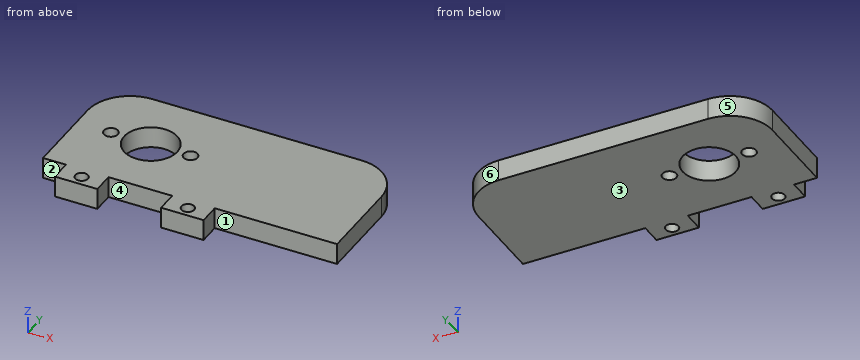
from build123d import *

# Parameters (mm, degrees)
SKETCH2_W                 = 87.884
SKETCH2_H                 = 44.45
BOSS_EXTRUDE1_DEPTH       = 3.175
CUT_EXTRUDE1_REACH        = 51.651
SKETCH3_R                 = 7.9375
F_8_CLEARANCE_HOLE1_D     = 4.1656
CIRPATTERN1_COUNT         = 2
CUT_EXTRUDE2_REACH        = 51.651
SKETCH6_W                 = 6.858
SKETCH6_H                 = 6.35
SKETCH6_W_2               = 19.05
SKETCH6_W_3               = 36.576
F_6_CLEARANCE_HOLE1_D     = 3.7973
F_6_CLEARANCE_HOLE1_DEPTH = 6.35
F_6_CLEARANCE_HOLE1_TIP   = 1.140824014
FILLET1_R                 = 12.7


with BuildPart() as part:
    # Sketch2 → Boss-Extrude1 (new, symmetric)
    with BuildSketch(Plane.XY):
        Rectangle(SKETCH2_W, SKETCH2_H)
    extrude(amount=BOSS_EXTRUDE1_DEPTH, both=True)

    # Sketch3 → Cut-Extrude1 (cut, up to next)
    with BuildSketch(Plane.XY.offset(3.175), mode=Mode.PRIVATE) as cut_extrude1_sk1:
        with Locations((-21.717, 3.175)):
            Circle(SKETCH3_R)
    cut_extrude1_tool1 = extrude(cut_extrude1_sk1.sketch, amount=-CUT_EXTRUDE1_REACH, mode=Mode.PRIVATE) & part.part
    add(cut_extrude1_tool1.solids().sort_by_distance((-21.717, 3.175, 3.175))[0], mode=Mode.SUBTRACT)

    # #8 Clearance Hole1 (through all)
    with Locations(Plane.XY.offset(3.175)):
        with Locations((-33.6169, 3.175)):
            f_8_clearance_hole1 = Hole(F_8_CLEARANCE_HOLE1_D / 2)

    # CirPattern1: #8 Clearance Hole1 ×2 about axis
    cirpattern1_axis = Axis((-21.717, 3.175, 0), (0, 0, 1))
    for i in range(1, CIRPATTERN1_COUNT):
        add(f_8_clearance_hole1.rotate(cirpattern1_axis, i * 360 / CIRPATTERN1_COUNT), mode=Mode.SUBTRACT)

    # Sketch6 → Cut-Extrude2 (cut, up to next)
    with BuildSketch(Plane.XY.offset(3.175), mode=Mode.PRIVATE) as cut_extrude2_sk1:
        with Locations((-40.513, -19.05)):
            Rectangle(SKETCH6_W, SKETCH6_H)
    cut_extrude2_tool1 = extrude(cut_extrude2_sk1.sketch, amount=-CUT_EXTRUDE2_REACH, mode=Mode.PRIVATE) & part.part
    # Sketch6 → Cut-Extrude2 (cut, up to next)
    with BuildSketch(Plane.XY.offset(3.175), mode=Mode.PRIVATE) as cut_extrude2_sk2:
        with Locations((-14.859, -19.05)):
            Rectangle(SKETCH6_W_2, SKETCH6_H)
    cut_extrude2_tool2 = extrude(cut_extrude2_sk2.sketch, amount=-CUT_EXTRUDE2_REACH, mode=Mode.PRIVATE) & part.part
    # Sketch6 → Cut-Extrude2 (cut, up to next)
    with BuildSketch(Plane.XY.offset(3.175), mode=Mode.PRIVATE) as cut_extrude2_sk3:
        with Locations((25.654, -19.05)):
            Rectangle(SKETCH6_W_3, SKETCH6_H)
    cut_extrude2_tool3 = extrude(cut_extrude2_sk3.sketch, amount=-CUT_EXTRUDE2_REACH, mode=Mode.PRIVATE) & part.part
    add(cut_extrude2_tool1.solids().sort_by_distance((-40.513, -19.05, 3.175))[0], mode=Mode.SUBTRACT)
    add(cut_extrude2_tool2.solids().sort_by_distance((-14.859, -19.05, 3.175))[0], mode=Mode.SUBTRACT)
    add(cut_extrude2_tool3.solids().sort_by_distance((25.654, -19.05, 3.175))[0], mode=Mode.SUBTRACT)

    # #6 Clearance Hole1
    with Locations(Plane.XY.offset(3.175)):
        with Locations((1.016, -19.05), (-30.734, -19.05)):
            Hole(F_6_CLEARANCE_HOLE1_D / 2, depth=F_6_CLEARANCE_HOLE1_DEPTH)
            with Locations((0, 0, -(F_6_CLEARANCE_HOLE1_DEPTH + F_6_CLEARANCE_HOLE1_TIP / 2))):  # 118° drill point
                Cone(0, F_6_CLEARANCE_HOLE1_D / 2, F_6_CLEARANCE_HOLE1_TIP, mode=Mode.SUBTRACT)

    # Fillet1
    fillet1_edges = [part.edges().sort_by_distance(p)[0] for p in [
        (-43.942, 22.225, 0),
        (43.942, 22.225, 0),
    ]]
    fillet(fillet1_edges, radius=FILLET1_R)


solid = part.part
Geometry: final body of the model. Coordinates: model frame, mm. Face numbers are marked on the shaded views. A direction names the side the tool comes from. Give positions to 0.01 mm unless a question says otherwise; leave off trailing zeros. Order: outer loops, then holes, each group sorted by start corner. A loop starts at its lowest first (then second) coordinate and runs counter-clockwise, first axis right, second up. Notation, with made-up numbers: (-9.5, -23.75) -> (-3.5, -23.75) arc R27 ccw to (-3.5, -4.75) -> close; hole circle Ø9 at (43.5, 69.25). An arc over 180 degrees is marked (long way). Put each result on its own line as item: value.
Q1. Reachability of the marked faces 1, 2 and 3 from +Z, -Z, +X, -X, +Y, -Y: full face, straight path, thin tool, end or side. Return the list, or none.
Here are the results:
face 1: +Z, -Z, +X, -Y
face 2: +Z, -Z, -X, -Y
face 3: -Z, +X, -X, +Y, -Y
Q2. Section C-C, the plane x = -18.5. Return loops of the section in (y, z) (3 decimals).
Here are the results:
outline: (-15.875, -3.175) -> (-4.081, -3.175) -> (-4.081, 3.175) -> (-15.875, 3.175) -> close; (10.431, -3.175) -> (22.225, -3.175) -> (22.225, 3.175) -> (10.431, 3.175) -> close
Q3. Material intervals for L1, parallel to X at y = 3, z = -1; L2, parallel to X at y = -19.05, z = 2; L3, parallel to X at y = -16.5, z = 0.25, sorted ascending.
Here are the results:
L1: x = -43.94 to -35.69, -31.54 to -29.65, -13.78 to -11.89, -7.74 to 43.94
L2: x = -37.08 to -32.63, -28.84 to -24.38, -5.33 to -0.88, 2.91 to 7.37
L3: x = -37.08 to -24.38, -5.33 to 7.37
Q4. Draft query along X for the marked faces 4, 5 and 6. Return one class per face: released by +X, released by -X, zero draft, split by the parting line, or undercut.
Here are the results:
face 4: undercut
face 5: released by -X
face 6: released by +X
Q5. Section D-D, the plane x = 24.5. Return loops of the section in (y, z) (3 decimals).
Here are the results:
outline: (-15.875, -3.175) -> (22.225, -3.175) -> (22.225, 3.175) -> (-15.875, 3.175) -> close
Q6. Section B-B, the plane z = -1.5. Count the separate pieces of the cut face and the enclosed holes in it, then the cut area to 3 significant figures.
Here are the results:
separate pieces: 1
enclosed holes: 5
area: 3,190 mm^2
Q7. Pin query (flat end, axial travel): pin 1 (1 mm diameter, centred on x = -18, z = 1, fed in from -Y) (3 decimals); pin 2 (1.5 mm diameter, centred on y = 13.5, z = -2, fed in from +X); pin 3 (3 mm diameter, centred on y = -19, z = -1.5, fed in from +X). Return the tip coordinate at first contact, or that it passes through.
Here are the results:
pin 1: stops at y = -15.875
pin 2: stops at x = 43.53
pin 3: stops at x = 7.37
Q8. Section A-A, the plane y = -19.05. Return loops of the section in (x, z) (3 decimals), then the cut area to 3 significant figures.
Here are the results:
outline: (-37.084, -3.175) -> (-32.633, -3.175) -> (-32.633, 3.175) -> (-37.084, 3.175) -> close; (-28.835, -3.175) -> (-24.384, -3.175) -> (-24.384, 3.175) -> (-28.835, 3.175) -> close; (-5.334, -3.175) -> (-0.883, -3.175) -> (-0.883, 3.175) -> (-5.334, 3.175) -> close; (2.915, -3.175) -> (7.366, -3.175) -> (7.366, 3.175) -> (2.915, 3.175) -> close
area: 113 mm^2
